Source: CAD feature listing. Evaluate the final solid. Frame: model axes, mm. A direction names the side the tool comes from. Coordinates: 2 decimals unless noted, no trailing zeros. Write each loop counter-clockwise with the first axis right and the second up, starting at its lowest first coordinate (ties: lowest second). Pieces come first, ordered by that corner, then holes. Notation, with made-up numbers: (79, 84) - (113, 84) arc R15 cw to (113, 98) - close; hole circle Ø7 at (-15.75, 70). An arc over 180 degrees is marked (long way). One line per question, with ' | ' between items. Start each with the question number.
Q1. Line query: line 1 (Y direction, x = 0, z = 4.95); line 2 (X direction, y = 19.5, z = 0); line 3 (Y direction, x = -1, z = 5.5). Output: solid intervals per line, ascending.
Q2. Cut plane B-B, the plane z = 0. Return loops of the section in (x, y), plus the area to 3 significant figures.
Q3. Access query for faces 4 (the face through (-0.339, 5.272, 4.784)), 5 (the face through (0, 18, 2.18)), 6 (the face through (0, 12.35, 3)). Directions: +Z, -Z, +X, -X, +Y, -Y. A direction counts if a zero-diameter tool reaches every point of the face in a straight line with its end or side. Return the directions, or none.
Q4. Contact query for flat-ended pins moving along their axis: P1, Ø3, axis at x = 0, y = 18.35, coming from the +Z side; P2, Ø2.5, axis at x = -1.5, z = -0.5, coming from the -Y side; P3, Ø6, axis at y = 15.5, z = -4, coming from the -X side; P4, Ø2, axis at y = 19, z = -2.5, coming from the -X side. Output: stop coordinate, or through.
Q5. Cut plane C-C, the plane y = 11. Return loops of the section in (x, z), plus the area to 3 significant figures.
Q6. Cut plane D-D, the plane x = 2. Return loops of the section in (y, z), plus the area to 3 significant figures.
Q7. Cut plane A-A, the plane x = 0. Return loops of the section in (y, z).
Q8. Draft query along Z for faces 1 (the face through (-1.3, 6.1, 3.26)), 2 (the face through (-3.86, 12.18, -5.04)), 3 (the face through (0, 0, 4)). Return one class per face: +Z half, -Z half, draft (parallel to the pull), parting line (faces both ways), or undercut.
```python
from build123d import *

# Parameters (mm, degrees)
SKETCH1_R           = 6.35
BOSS_EXTRUDE1_DEPTH = 12.35
SKETCH4_R           = 6.35
BOSS_EXTRUDE2_DEPTH = 12.35
SKETCH5_R           = 1.13
CUT_EXTRUDE2_DEPTH  = 28.253825364


with BuildPart() as part:
    # Sketch1 → Boss-Extrude1 (new body)
    with BuildSketch(Plane(origin=(0, 0, 0), x_dir=(1, 0, 0), z_dir=(0, 1, 0))):
        with Locations(Location((0, 0, 0), (0, 0, 270))):
            Circle(SKETCH1_R)
        with BuildLine():
            Line((-2.742383206, -3.260332823), (2.742383206, -3.260332823))
            ThreePointArc((2.742383206, -3.260332823), (0, 4.260332823), (-2.742383206, -3.260332823))
        make_face(mode=Mode.SUBTRACT)
    extrude(amount=BOSS_EXTRUDE1_DEPTH)

    # Sketch4 → Boss-Extrude2 (add)
    with BuildSketch(Plane(origin=(0, 12.35, 0), x_dir=(1, 0, 0), z_dir=(0, 1, 0))):
        with Locations(Location((0, 0, 0), (0, 0, 270))):
            Circle(SKETCH4_R)
        with BuildLine():
            Line((-2.315167381, -2.18), (2.315167381, -2.18))
            ThreePointArc((2.315167381, -2.18), (0, 3.18), (-2.315167381, -2.18))
        make_face(mode=Mode.SUBTRACT)
    extrude(amount=BOSS_EXTRUDE2_DEPTH)

    # Sketch5 → Cut-Extrude2 (cut, through all)
    with BuildSketch(Plane(origin=(0, 0, 3.260332823), x_dir=(-1, 0, 0), z_dir=(0, 0, -1))):
        with Locations((0, 18.35)):
            Circle(SKETCH5_R)
        with Locations(Location((0, 6.35, 0), (0, 0, 270))):
            Circle(SKETCH5_R)
    extrude(amount=-CUT_EXTRUDE2_DEPTH, mode=Mode.SUBTRACT)


solid = part.part
```
Reply:
1) line 1: y = 0 to 5.22, 7.48 to 17.22, 19.48 to 24.7 | line 2: x = -6.35 to -3.18, 3.18 to 6.35 | line 3: y = 0 to 5.82, 6.88 to 17.82, 18.88 to 24.7
2) outline: (-6.35, 0) - (-4.26, 0) - (-4.26, 12.35) - (-3.18, 12.35) - (-3.18, 24.7) - (-6.35, 24.7) - close; (3.18, 12.35) - (4.26, 12.35) - (4.26, 0) - (6.35, 0) - (6.35, 24.7) - (3.18, 24.7) - close | area: 130 mm^2
3) face 4: +Z | face 5: +Y, -Y | face 6: -Y
4) P1: stops at z = 6.35 | P2: passes through | P3: stops at x = -6.27 | P4: stops at x = -6.17
5) outline: circle Ø12.7 at (0, 0); hole (-2.74, 3.26) arc R4.26 ccw (long way) to (2.74, 3.26) - close | area: 73.4 mm^2
6) outline: (0, -6.03) - (24.7, -6.03) - (24.7, -2.47) - (12.35, -2.47) - (12.35, -3.76) - (0, -3.76) - close; (0, 3.26) - (12.35, 3.26) - (12.35, 2.18) - (24.7, 2.18) - (24.7, 6.03) - (0, 6.03) - close | area: 154 mm^2
7) outline: (0, -6.35) - (24.7, -6.35) - (24.7, -3.18) - (12.35, -3.18) - (12.35, -4.26) - (0, -4.26) - close; (0, 3.26) - (5.22, 3.26) - (5.22, 6.35) - (0, 6.35) - close; (7.48, 3.26) - (12.35, 3.26) - (12.35, 2.18) - (24.7, 2.18) - (24.7, 6.35) - (19.48, 6.35) - (19.48, 3.26) - (17.22, 3.26) - (17.22, 6.35) - (7.48, 6.35) - close
8) face 1: undercut | face 2: parting line | face 3: draft
